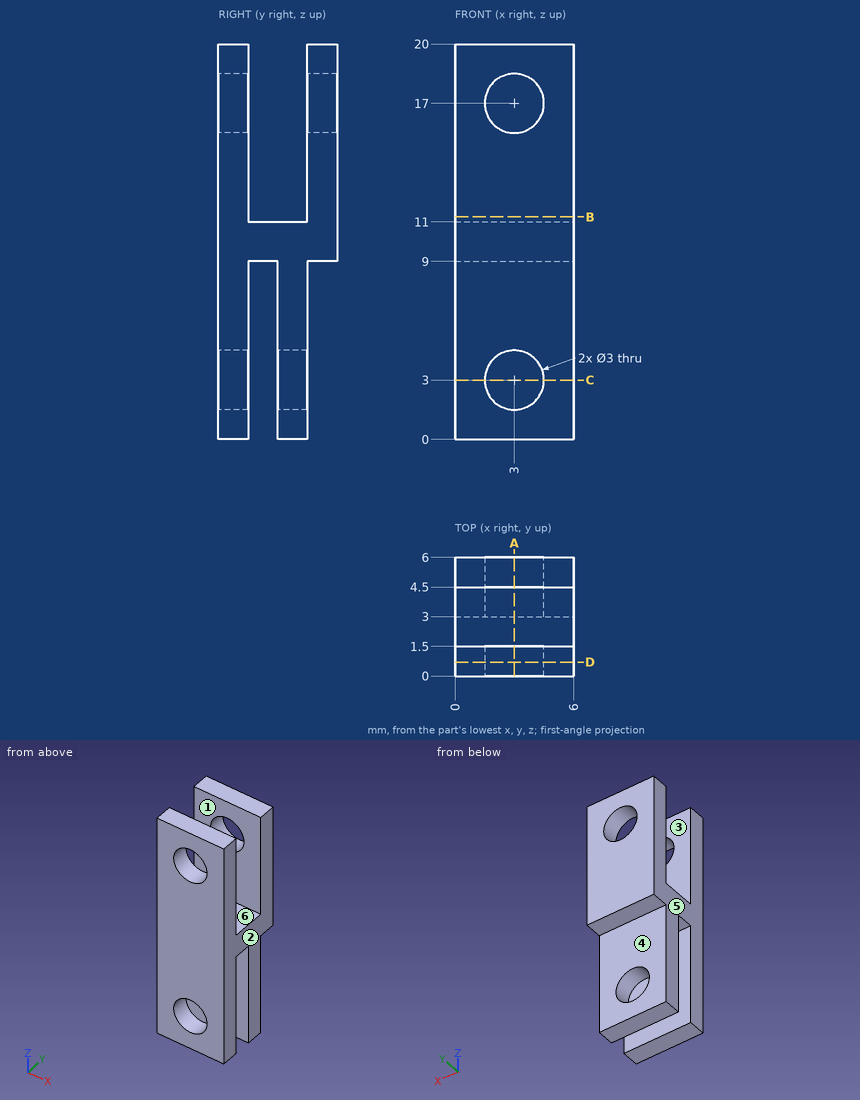
Could you check a few things on this drawing? It's one solid part, dimensions in mm from its lowest x, y, z. A direction names the side the tool comes from. Coordinates: 2 decimals unless noted, no trailing zeros. Order: outer loops, then holes, each group sorted by start corner. A loop starts at its lowest first (then second) coordinate and runs counter-clockwise, first axis right, second up. Notation, with made-up numbers: M 35,20 L 42,20 A8 cw 42,28 Z; hole C 45,41 d4. An arc over 180 degrees is marked long. Answer as a JSON object with one key per item and string values. Group by question number.
(1) I need wall thicknesses on probe 1 along Z at (x, y) = (3, 0.8); probe 2 along Y at (x, z) = (3.65, 12); probe 3 along Y at (x, z) = (3.5, 8). Which ranges of each line are inside material? Lowest first, please.
(2) Suppose I cut it at D-D, the plane y = 0.7. Please give me the cut outline in (x, z).
(3) Suppose I cut it at C-C, the plane z = 3. Please give me the cut outline in (x, y).
(4) If we mould it in two halves opening along Y, with no side actions, what happens to the marked faces 1, 2, 3 and 4? For each: released by +Y, released by -Y, zero draft, split by the parting line, or undercut.
(5) Suppose I cut it at A-A, the plane x = 3. State how many separate pieces and enclosed holes the cut face has, then the cut area to 3 significant figures.
(6) Which directions (+Z, -Z, +X, -X, +Y, -Y) give clear straight access to the entire face, cutting with the end or side of a thin tool? Please do the marked faces 5 and 6.
(7) For pin 1 (1.5 mm diameter, centred on x = 2.5, y = 2.5, fed in from +Z); pin 2 (2.5 mm diameter, centred on x = 3, z = 17, fed in from +Y); pin 3 (0.8 mm diameter, centred on x = 3.5, y = 2.5, fed in from -Z); pin 4 (3 mm diameter, centred on x = 2.5, z = 6, fed in from +Y), each with a flat end and sliding along its axis, tell me the tip position at first contact or that it passes through.
(8) Suppose I cut it at B-B, the plane z = 11.25. Please give me the cut outline in (x, y), then the cut area to 3 significant figures.
Values found:
{
 "1": {"probe 1": "z = 0 to 1.5, 4.5 to 15.5, 18.5 to 20", "probe 2": "y = 0 to 1.5, 4.5 to 6", "probe 3": "y = 0 to 1.5, 3 to 4.5"},
 "2": {"outline": "M 0,0 L 6,0 L 6,20 L 0,20 Z; hole C 3,3 d3; hole C 3,17 d3"},
 "3": {"outline": "M 0,0 L 1.5,0 L 1.5,1.5 L 0,1.5 Z; M 0,3 L 1.5,3 L 1.5,4.5 L 0,4.5 Z; M 4.5,0 L 6,0 L 6,1.5 L 4.5,1.5 Z; M 4.5,3 L 6,3 L 6,4.5 L 4.5,4.5 Z"},
 "4": {"face 1": "undercut", "face 2": "zero draft", "face 3": "undercut", "face 4": "released by +Y"},
 "5": {"separate pieces": "5", "enclosed holes": "0", "area": "48.0 mm^2"},
 "6": {"face 5": "+Z, -Z, -X, +Y, -Y", "face 6": "+Z, +X, -X"},
 "7": {"pin 1": "stops at z = 11", "pin 2": "passes through", "pin 3": "stops at z = 9", "pin 4": "stops at y = 4.5"},
 "8": {"outline": "M 0,0 L 6,0 L 6,1.5 L 0,1.5 Z; M 0,4.5 L 6,4.5 L 6,6 L 0,6 Z", "area": "18.0 mm^2"}
}
